The model under review builds one solid part; all positions refer to its coordinate system, in mm. Face numbers are marked on the shaded views. A direction names the side the tool comes from. Coordinates: 2 decimals unless noted, no trailing zeros. Order: outer loops, then holes, each group sorted by start corner. A loop starts at its lowest first (then second) coordinate and runs counter-clockwise, first axis right, second up. Notation, with made-up numbers: (65.25, -23.75) -> (109.25, -23.75) arc R26 ccw to (109.25, -4.75) -> close; hole circle Ø4 at (66.25, 41.5). An arc over 180 degrees is marked (long way). Use one line per item in the form item = value.
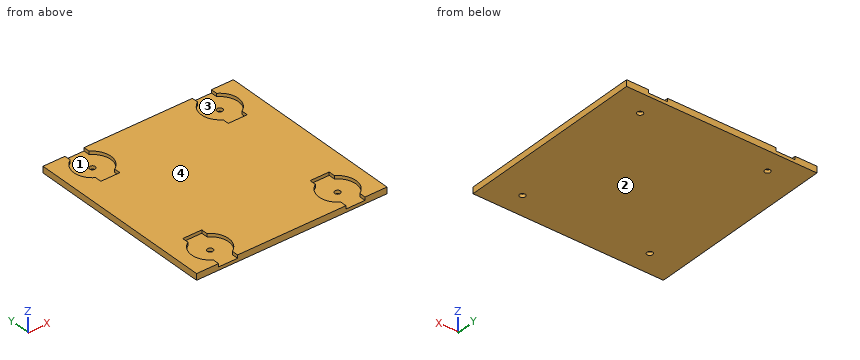
from build123d import *

# Parameters (mm, degrees)
SKETCH_W        = 60
SKETCH_H        = 60
PAD_DEPTH       = 2
POCKET001_DEPTH = 1
SKETCH005_R     = 0.9
POCKET002_DEPTH = 5


with BuildPart() as part:
    # Sketch → Pad (new body)
    with BuildSketch(Plane.XY):
        Rectangle(SKETCH_W, SKETCH_H)
    extrude(amount=PAD_DEPTH)

    # Sketch004 (on Face6 of Pad) → Pocket001 (cut)
    with BuildSketch(Plane.XY.offset(2)):
        with BuildLine():
            Line((-23.070984, -27.963869), (-23.070984, -30))
            Line((-23.070984, -30), (-17.070984, -30))
            Line((-17.070984, -30), (-17.070984, -27.963869))
            ThreePointArc((-17.070984, -27.963869), (-14.270984, -23), (-17.070984, -18.036131))
            Line((-17.070984, -16), (-17.070984, -18.036131))
            Line((-23.070984, -16), (-17.070984, -16))
            Line((-23.070984, -18.036131), (-23.070984, -16))
            ThreePointArc((-23.070984, -18.036131), (-25.870984, -23), (-23.070984, -27.963869))
        make_face()
        with BuildLine():
            Line((23.070984, -27.963869), (23.070984, -30))
            Line((23.070984, -30), (17.070984, -30))
            Line((17.070984, -30), (17.070984, -27.963869))
            ThreePointArc((17.070984, -18.036131), (14.270984, -23), (17.070984, -27.963869))
            Line((17.070984, -16), (17.070984, -18.036131))
            Line((23.070984, -16), (17.070984, -16))
            Line((23.070984, -18.036131), (23.070984, -16))
            ThreePointArc((23.070984, -27.963869), (25.870984, -23), (23.070984, -18.036131))
        make_face()
        with BuildLine():
            Line((-23.070984, 27.963869), (-23.070984, 30))
            Line((-23.070984, 30), (-17.070984, 30))
            Line((-17.070984, 30), (-17.070984, 27.963869))
            ThreePointArc((-17.070984, 18.036131), (-14.270984, 23), (-17.070984, 27.963869))
            Line((-17.070984, 16), (-17.070984, 18.036131))
            Line((-23.070984, 16), (-17.070984, 16))
            Line((-23.070984, 18.036131), (-23.070984, 16))
            ThreePointArc((-23.070984, 27.963869), (-25.870984, 23), (-23.070984, 18.036131))
        make_face()
        with BuildLine():
            Line((23.070984, 27.963869), (23.070984, 30))
            Line((23.070984, 30), (17.070984, 30))
            Line((17.070984, 30), (17.070984, 27.963869))
            ThreePointArc((17.070984, 27.963869), (14.270984, 23), (17.070984, 18.036131))
            Line((17.070984, 16), (17.070984, 18.036131))
            Line((23.070984, 16), (17.070984, 16))
            Line((23.070984, 18.036131), (23.070984, 16))
            ThreePointArc((23.070984, 18.036131), (25.870984, 23), (23.070984, 27.963869))
        make_face()
    extrude(amount=-POCKET001_DEPTH, mode=Mode.SUBTRACT)

    # Sketch005 (on Face4 of Pocket001) → Pocket002 (cut)
    with BuildSketch(Plane.XY.offset(2)):
        with Locations((-20.070984, -23)):
            Circle(SKETCH005_R)
        with Locations((20.070984, -23)):
            Circle(SKETCH005_R)
        with Locations((-20.070984, 23)):
            Circle(SKETCH005_R)
        with Locations((20.070984, 23)):
            Circle(SKETCH005_R)
    extrude(amount=-POCKET002_DEPTH, mode=Mode.SUBTRACT)


solid = part.part
Item 1: Clearance check with a flat-ended pin moving along its axis: pin 1 (3.5 mm diameter, centred on x = -19.5, y = -20.5, fed in from +Z). State where the tip first meets the part, or that it passes through.
Results found:
pin_1 = 1
Item 2: Tool access review of the marked faces 1 and 2: name each direction out of +Z, -Z, +X, -X, +Y, -Y from which nothing blocks a thin tool from reaching the whole face with its end or side.
Results found:
face_1 = +Z
face_2 = -Z, +X, -X, +Y, -Y
Item 3: Draft analysis for pull direction X (two halves, no side actions). For the marked faces 3 and 4, state which applies: released by +X, released by -X, zero draft, split by the parting line, or undercut.
Results found:
face_3 = undercut
face_4 = zero draft
Item 4: We need section B-B (x = 15.5). Write out the cut boundary in (y, z).
Results found:
outline = (-30, 0) -> (30, 0) -> (30, 2) -> (26.57, 2) -> (26.57, 1) -> (19.43, 1) -> (19.43, 2) -> (-19.43, 2) -> (-19.43, 1) -> (-26.57, 1) -> (-26.57, 2) -> (-30, 2) -> close
Item 5: We need section A-A (y = 23). Write out the cut boundary in (x, z).
Results found:
outline = (-30, 0) -> (-20.97, 0) -> (-20.97, 1) -> (-25.87, 1) -> (-25.87, 2) -> (-30, 2) -> close; (-19.17, 0) -> (19.17, 0) -> (19.17, 1) -> (14.27, 1) -> (14.27, 2) -> (-14.27, 2) -> (-14.27, 1) -> (-19.17, 1) -> close; (20.97, 0) -> (30, 0) -> (30, 2) -> (25.87, 2) -> (25.87, 1) -> (20.97, 1) -> close
Item 6: To check wall thickness, follow L1, parallel to Y at x = 19.5, z = 0.45; L2, parallel to Z at x = 23, y = -20.5; L3, parallel to Y at x = 20.5, z = 1.1. State the ranges of each line that lie inside material, in increasing order. Write a range as from..to.
Results found:
L1 = -30..-23.7, -22.3..22.3, 23.7..30
L2 = 0..1
L3 = -16..16
